Read the model definition and answer for the solid it produces. Units are mm, in the model's axes. A direction names the side the tool comes from. Coordinates: 2 decimals unless noted, no trailing zeros. Write each loop counter-clockwise with the first axis right and the second up, starting at its lowest first coordinate (ties: lowest second). Pieces come first, ordered by that corner, then holes.
(1) Determine the mould class of faces 1 (the flat face through (5.69, -17.24, 10.5)), 2 (the cylindrical face through (-2.343, 17.847, 5.937)), 3 (the cylindrical face through (-2.539, 19.334, 0.74)), 4 (the flat face through (0, -4, 12)) for opening direction Z: pulls with the +Z half, pulls with the -Z half, needs draft (parallel to the pull), parting line crosses it, or undercut.
(2) The part is cut by section D-D, the plane y = -10. Determine the outline of the cut face in (x, z).
(3) Straight lines are drawn through the part: line 1 along Z through (x, y) = (-5, 18); line 2 along Y through (x, z) = (0, 3); line 3 along X through (y, z) = (-7, 11.25). For each, find the intervals that lie inside material, in ascending order.
(4) Which of the six approach directions +Z, -Z, +X, -X, +Y, -Y give full straight-line access (tool end or side, diameter ignored) to faces 5 (the flat face through (5.69, -17.24, 1.5)), 6 (the cylindrical face through (-2.539, 19.334, 11.24))?
(5) Given pin 1 (2 mm diameter, centred on x = -11.5, z = 4.5, fed in from -Y); pin 2 (1.5 mm diameter, centred on x = 4, z = 10, fed in from -Y); pin 3 (1.5 mm diameter, centred on y = 8.5, z = 3.5, fed in from -X), each flat-ended and moving along its own axis, determine where each tip first touches the part or whether it passes through.
(6) The part is cut by section C-C, the plane z = 6.75. Determine the outline of the cut face in (x, y).
(7) The part is cut by section A-A, the plane y = 0. Determine the outline of the cut face in (x, z).
```python
from build123d import *

# Parameters (mm, degrees)
SKETCH_1_R               = 19.5
EXTRUDE_1_DEPTH          = 12
CUT_EXTRUDE_1_DEPTH      = 4.5
CUT_EXTRUDE_1_DEPTH_BACK = 4.5
SKETCH_2_R               = 19.5
SKETCH_2_R_2             = 18
SKETCH_3_R               = 3
CUT_EXTRUDE_2_DEPTH      = 31.074906484


with BuildPart() as part:
    # 草图1 → 凸台-拉伸1 (new body)
    with BuildSketch(Plane.XY):
        Circle(SKETCH_1_R)
    extrude(amount=EXTRUDE_1_DEPTH)

    # 草图2 → 切除-拉伸1 (cut, two sides: drawn at the far end of the back side and taken through both)
    with BuildSketch(Plane.XY.offset(6).offset(-CUT_EXTRUDE_1_DEPTH_BACK)):
        Circle(SKETCH_2_R)
        Circle(SKETCH_2_R_2, mode=Mode.SUBTRACT)
    extrude(amount=CUT_EXTRUDE_1_DEPTH + CUT_EXTRUDE_1_DEPTH_BACK, mode=Mode.SUBTRACT)

    # 草图3 → 切除-拉伸2 (cut, through all)
    with BuildSketch(Plane.XY.offset(12)):
        Circle(SKETCH_3_R)
    extrude(amount=-CUT_EXTRUDE_2_DEPTH, mode=Mode.SUBTRACT)


solid = part.part
```
Computed:
1. face 1: undercut
1. face 2: undercut
1. face 3: needs draft
1. face 4: pulls with the +Z half
2. outline: (-16.74, 0) - (16.74, 0) - (16.74, 1.5) - (14.97, 1.5) - (14.97, 10.5) - (16.74, 10.5) - (16.74, 12) - (-16.74, 12) - (-16.74, 10.5) - (-14.97, 10.5) - (-14.97, 1.5) - (-16.74, 1.5) - close
3. line 1: z = 0 to 1.5, 10.5 to 12
3. line 2: y = -18 to -3, 3 to 18
3. line 3: x = -18.2 to 18.2
4. face 5: none
4. face 6: +Z, -Z
5. pin 1: stops at y = -14.62
5. pin 2: stops at y = -19.19
5. pin 3: stops at x = -16.25
6. outline: circle Ø36 at (0, 0); hole circle Ø6 at (0, 0)
7. outline: (-19.5, 0) - (-3, 0) - (-3, 12) - (-19.5, 12) - (-19.5, 10.5) - (-18, 10.5) - (-18, 1.5) - (-19.5, 1.5) - close; (3, 0) - (19.5, 0) - (19.5, 1.5) - (18, 1.5) - (18, 10.5) - (19.5, 10.5) - (19.5, 12) - (3, 12) - close
